```python
from build123d import *

# Parameters (mm, degrees)
SKETCH1_R           = 50
BOSS_EXTRUDE1_DEPTH = 221.459907
SKETCH2_R           = 27.18721444
CUT_EXTRUDE1_DEPTH  = 233.47470918
CHAMFER1_SIZE       = 3.603241


with BuildPart() as part:
    # Sketch1 → Boss-Extrude1 (new body)
    with BuildSketch(Plane(origin=(0, 0, 0), x_dir=(1, 0, 0), z_dir=(0, 1, 0))):
        with Locations(Location((0, 0, 0), (0, 0, 90))):
            Circle(SKETCH1_R)
    extrude(amount=BOSS_EXTRUDE1_DEPTH)

    # Sketch2 → Cut-Extrude1 (cut, through all)
    with BuildSketch(Plane(origin=(0, 0, 0), x_dir=(1, 0, 0), z_dir=(0, 1, 0))):
        with Locations(Location((0, 0, 0), (0, 0, 90))):
            Circle(SKETCH2_R)
    extrude(amount=CUT_EXTRUDE1_DEPTH, mode=Mode.SUBTRACT)

    # Chamfer1
    chamfer1_edges = [part.edges().sort_by_distance(p)[0] for p in [
        (0, 0, 50),
        (0, 221.459907, 50),
        (0, 0, 27.18721444),
        (0, 221.459907, 27.18721444),
    ]]
    chamfer(chamfer1_edges, length=CHAMFER1_SIZE)


solid = part.part
```
Source: CAD feature listing. Evaluate the final solid. Frame: model axes, mm. Round coordinates to 2 decimals unless told otherwise and drop trailing zeros. Loops run counter-clockwise (first coordinate to the right, second up) from the corner with the lowest first, then second, coordinate; pieces in that order, holes last.
1. Contact query for flat-ended pins moving along their axis: pin 1 (4 mm diameter, centred on x = 31, y = 37.5, fed in from -Z); pin 2 (1 mm diameter, centred on x = 13, z = 32, fed in from -Y); pin 3 (3 mm diameter, centred on x = 22.5, y = 131, fed in from +Z); pin 4 (8 mm diameter, centred on y = 40.5, z = 36, fed in from +X). Output: stop coordinate, or through.
2. Section query A-A on x = 0. Output: boundary loops of the cut face in (y, z), and give its area (3 significant figures).
3. Ray query, L1, parallel to X at y = 63, z = 0; L2, parallel to Z at x = -7, y = 122; L3, parallel to Z at x = -15, y = 170.5. Return the intervals inside material, ascending.
4. Section query C-C on y = 135.5. Output: boundary loops of the cut face in (x, z).
5. Section query B-B on z = 0. Output: boundary loops of the cut face in (x, y).
6. Mould query, pull axis Z, two halves, no side actions, for faces 1 (the conical face through (28.34, 221.28, 36.96)), 2 (the flat face through (10, 0, -30)), 3 (the conical face through (-26.71, 218.03, 5.93)). Classes: released by +Z, released by -Z, zero draft, split by the parting line, or undercut.
Answers below:
1. pin 1: stops at z = -40.73
1. pin 2: stops at y = 0
1. pin 3: stops at z = 45.38
1. pin 4: stops at x = 38.42
2. outline: (0, -46.4) - (3.6, -50) - (217.86, -50) - (221.46, -46.4) - (221.46, -30.79) - (217.86, -27.19) - (3.6, -27.19) - (0, -30.79) - close; (0, 30.79) - (3.6, 27.19) - (217.86, 27.19) - (221.46, 30.79) - (221.46, 46.4) - (217.86, 50) - (3.6, 50) - (0, 46.4) - close
2. area: 10,100 mm2
3. L1: x = -50 to -27.19, 27.19 to 50
3. L2: z = -49.51 to -26.27, 26.27 to 49.51
3. L3: z = -47.7 to -22.67, 22.67 to 47.7
4. outline: circle Ø100 at (0, 0); hole circle Ø54.37 at (0, 0)
5. outline: (-50, 3.6) - (-46.4, 0) - (-30.79, 0) - (-27.19, 3.6) - (-27.19, 217.86) - (-30.79, 221.46) - (-46.4, 221.46) - (-50, 217.86) - close; (27.19, 3.6) - (30.79, 0) - (46.4, 0) - (50, 3.6) - (50, 217.86) - (46.4, 221.46) - (30.79, 221.46) - (27.19, 217.86) - close
6. face 1: split by the parting line
6. face 2: zero draft
6. face 3: undercut
